Geometry: final body of the model. Coordinates: model frame, mm. A direction names the side the tool comes from. Give positions to 0.01 mm unless a question says otherwise; leave off trailing zeros. Order: outer loops, then holes, each group sorted by start corner. A loop starts at its lowest first (then second) coordinate and runs counter-clockwise, first axis right, second up. Notation, with made-up numbers: (-28, 80) -> (-3, 80) arc R26 ccw to (-3, 107) -> close; hole circle Ø5 at (17.5, 14). An arc over 180 degrees is marked (long way). Write item = value, one per line.
```python
from build123d import *

# Parameters (mm, degrees)
CROQUIS1_R              = 1.25
SALIENTE_EXTRUIR1_DEPTH = 2
SALIENTE_EXTRUIR2_DEPTH = 71.5


with BuildPart() as part:
    # Croquis1 → Saliente-Extruir1 (new body)
    with BuildSketch(Plane(origin=(0, 0, 0), x_dir=(1, 0, 0), z_dir=(0, 1, 0))):
        with BuildLine():
            Line((36.224750286, -45.279704968), (34.517643505, -43.572598187))
            Line((34.517643505, -43.572598187), (34.517643505, -15.751506533))
            ThreePointArc((34.517643505, -15.751506533), (24.517643505, 1.427401813), (14.517643505, -15.751506533))
            Line((14.517643505, -15.751506533), (14.517643505, -43.572598187))
            Line((14.517643505, -43.572598187), (12.810536723, -45.279704968))
            ThreePointArc((12.810536723, -45.279704968), (12.486113375, -45.49647772), (12.103429942, -45.572598187))
            Line((12.103429942, -45.572598187), (8.017643505, -45.572598187))
            ThreePointArc((8.017643505, -45.572598187), (7.310536723, -45.279704968), (7.017643505, -44.572598187))
            Line((7.017643505, -44.572598187), (7.017643505, -36.572598187))
            Line((7.017643505, -36.572598187), (-2.482356495, -28.572598187))
            Line((-2.482356495, -28.572598187), (-11.232356495, -28.572598187))
            Line((-11.232356495, -28.572598187), (-11.232356495, 8.427401813))
            Line((-11.232356495, 8.427401813), (60.267643505, 8.427401813))
            Line((60.267643505, 8.427401813), (60.267643505, -28.572598187))
            Line((60.267643505, -28.572598187), (51.517643505, -28.572598187))
            Line((51.517643505, -28.572598187), (42.017643505, -36.572598187))
            Line((42.017643505, -36.572598187), (42.017643505, -44.572598187))
            ThreePointArc((42.017643505, -44.572598187), (41.724750286, -45.279704968), (41.017643505, -45.572598187))
            Line((41.017643505, -45.572598187), (36.931857067, -45.572598187))
            ThreePointArc((36.931857067, -45.572598187), (36.549173635, -45.49647772), (36.224750286, -45.279704968))
        make_face()
        with Locations(Location((37.017643505, -18.072598187, 0), (0, 0, 90))):
            Circle(CROQUIS1_R, mode=Mode.SUBTRACT)
        with Locations(Location((36.517643505, -41.572598187, 0), (0, 0, 90))):
            Circle(CROQUIS1_R, mode=Mode.SUBTRACT)
        with Locations(Location((12.517643505, -41.572598187, 0), (0, 0, 270))):
            Circle(CROQUIS1_R, mode=Mode.SUBTRACT)
        with Locations(Location((12.017643505, -18.072598187, 0), (0, 0, 270))):
            Circle(CROQUIS1_R, mode=Mode.SUBTRACT)
    extrude(amount=-SALIENTE_EXTRUIR1_DEPTH)

    # Croquis3 → Saliente-Extruir2 (add)
    with BuildSketch(Plane(origin=(60.267643505, 0, 0), x_dir=(0, 0, -1), z_dir=(1, 0, 0))):
        Polygon((-25.572598187, 0), (-25.572598187, 4.5), (-29.572598187, 4.5), (-29.572598187, 2.5), (-27.572598187, 2.5), (-27.572598187, 1), (-28.572598187, 1), (-28.572598187, 0), align=None)
        Polygon((5.427401813, 4.5), (9.427401813, 4.5), (9.427401813, 2.5), (7.427401813, 2.5), (7.427401813, 1), (8.427401813, 1), (8.427401813, 0), (5.427401813, 0), align=None)
    extrude(amount=-SALIENTE_EXTRUIR2_DEPTH)


solid = part.part
```
1) Section query A-A (z = 21.5). Output: boundary loops of the cut face in (x, y).
Check sheet entries:
outline = (-11.23, -2) -> (14.52, -2) -> (14.52, 0) -> (-11.23, 0) -> close; (34.52, -2) -> (60.27, -2) -> (60.27, 0) -> (34.52, 0) -> close
2) Section query C-C (x = -3.5). Output: boundary loops of the cut face in (y, z).
Check sheet entries:
outline = (-2, -8.43) -> (1, -8.43) -> (1, -7.43) -> (2.5, -7.43) -> (2.5, -9.43) -> (4.5, -9.43) -> (4.5, -5.43) -> (0, -5.43) -> (0, 25.57) -> (4.5, 25.57) -> (4.5, 29.57) -> (2.5, 29.57) -> (2.5, 27.57) -> (1, 27.57) -> (1, 28.57) -> (-2, 28.57) -> close
3) Section query B-B (y = 3.5). Output: boundary loops of the cut face in (x, z), plus the area to 3 significant figures.
Check sheet entries:
outline = (-11.23, -9.43) -> (60.27, -9.43) -> (60.27, -5.43) -> (-11.23, -5.43) -> close; (-11.23, 25.57) -> (60.27, 25.57) -> (60.27, 29.57) -> (-11.23, 29.57) -> close
area = 572 mm²
4) Reachability of faces 1 (the face through (14.518, -1, 29)), 2 (the face through (25, 4, 29.573)), 3 (the face through (33, 0, 0)) from +Z, -Z, +X, -X, +Y, -Y: full face, straight path, thin tool, end or side. Return the list, or none.
Check sheet entries:
face_1 = +Z, -Y
face_2 = +Z, +X, -X, +Y
face_3 = +X, -X, +Y
5) Line query: line 1 (Z direction, x = 25, y = 1.5); line 2 (Z direction, x = 23, y = 0.25); line 3 (Y direction, x = 35.5, z = 29). Output: solid intervals per line, ascending. Write a range as from..to.
Check sheet entries:
line_1 = -7.43..-5.43, 25.57..27.57
line_2 = -8.43..-5.43, 25.57..28.57
line_3 = -2..0, 2.5..4.5
6) Mould query, pull axis Z, two halves, no side actions, for faces 4 (the face through (7.018, -1, 41)), 5 (the face through (25, 4, -9.427)), 6 (the face through (24.854, -0.986, -1.422)). Classes: +Z half, -Z half, draft (parallel to the pull), parting line (faces both ways), or undercut.
Check sheet entries:
face_4 = draft
face_5 = -Z half
face_6 = undercut
7) Section query D-D (x = 30). Output: boundary loops of the cut face in (y, z), plus the area to 3 significant figures.
Check sheet entries:
outline = (-2, -8.43) -> (1, -8.43) -> (1, -7.43) -> (2.5, -7.43) -> (2.5, -9.43) -> (4.5, -9.43) -> (4.5, -5.43) -> (0, -5.43) -> (0, -0.04) -> (-2, -0.04) -> close; (0, 25.57) -> (4.5, 25.57) -> (4.5, 29.57) -> (2.5, 29.57) -> (2.5, 27.57) -> (1, 27.57) -> (1, 28.57) -> (0, 28.57) -> close
area = 44.8 mm²
8) First-contact query: P1, Ø3, axis at x = 12.52, z = 41.57, coming from the +Y side; P2, Ø0.8, axis at x = 36, y = 2, coming from the -Z side; P3, Ø2, axis at y = -1, z = 42, coming from the +X side. Flat tips, straight axial feed; report the tip coordinate or a pass-through.
Check sheet entries:
P1 = 0
P2 = -7.43
P3 = 42.02
